Work out the finished part from the listing and answer in its coordinate system (mm). Give positions to 0.01 mm unless a question says otherwise; leave off trailing zeros. Order: outer loops, then holes, each group sorted by start corner. A loop starts at its lowest first (then second) coordinate and runs counter-clockwise, first axis right, second up. Notation, with made-up numbers: (-16.5, 82.5) -> (11.5, 82.5) arc R18 cw to (11.5, 106.5) -> close; hole circle Ø11 at (-8, 38). An arc over 180 degrees is marked (long way). Use a Markdown table: item, result. Add a question column.
```python
from build123d import *

# Parameters (mm, degrees)
SKETCH1_R           = 10
SKETCH1_R_2         = 1.972602619
BOSS_EXTRUDE2_DEPTH = 2
SKETCH5_W           = 5
SKETCH5_H           = 14
CUT_EXTRUDE3_DEPTH  = 3.0000001
SKETCH6_W           = 5
SKETCH6_H           = 14
CUT_EXTRUDE4_DEPTH  = 3.0000001
SKETCH19_R          = 2
CUT_EXTRUDE19_DEPTH = 3.0000001
SKETCH22_R          = 2
CUT_EXTRUDE22_DEPTH = 3.0000001
SKETCH23_R          = 2
CUT_EXTRUDE23_DEPTH = 3.0000001
SKETCH24_R          = 2
CUT_EXTRUDE24_DEPTH = 3.0000001
SKETCH25_W          = 5
SKETCH25_H          = 12
CUT_EXTRUDE25_DEPTH = 3.0000001
CUT_EXTRUDE26_DEPTH = 3.0000001
CUT_EXTRUDE29_DEPTH = 3.0000001
SKETCH20_R          = 2
CUT_EXTRUDE20_DEPTH = 3.0000001
SKETCH30_W          = 181.696441894
SKETCH30_H          = 131.456906608
CUT_EXTRUDE30_DEPTH = 3
SKETCH31_R          = 2
CUT_EXTRUDE31_DEPTH = 2
SKETCH32_W          = 167.461823271
SKETCH32_H          = 37.26795508
CUT_EXTRUDE32_DEPTH = 2
FILLET1_R           = 10
FILLET2_R           = 5


with BuildPart() as part:
    # Sketch1 → Boss-Extrude2 (new body)
    with BuildSketch(Plane.XY):
        with BuildLine():
            Line((-49.4, 97.775402254), (-49.4, 48.775402254))
            Line((-49.4, 48.775402254), (-48.4, 48.775402254))
            Line((-48.4, 48.775402254), (-48.4, 35.775402254))
            Line((-48.4, 35.775402254), (-49.4, 35.775402254))
            Line((-49.4, 35.775402254), (-49.4, 21.775402254))
            Line((-49.4, 21.775402254), (-73.4, 21.775402254))
            Line((-73.4, 21.775402254), (-73.4, -12.924597746))
            Line((-73.4, -12.924597746), (-49.4, -12.924597746))
            Line((-49.4, -12.924597746), (-49.4, -26.924597746))
            Line((-49.4, -26.924597746), (-48.4, -26.924597746))
            Line((-48.4, -26.924597746), (-48.4, -39.924597746))
            Line((-48.4, -39.924597746), (-49.4, -39.924597746))
            Line((-49.4, -39.924597746), (-49.4, -88.924597746))
            Line((-49.4, -88.924597746), (-73.349457369, -88.924597746))
            add(Edge.make_bspline(
                [(-73.349457369, -88.924597746), (-70.502213021, -123.490651401), (3.447241601, -123.490651401), (77.396696223, -123.490651401), (74.549451875, -88.924597746)],
                knots=[3.190793702, 3.190793702, 3.190793702, 4.761590029, 4.761590029, 6.332386355, 6.332386355, 6.332386355], degree=2, weights=[1, 0.707106781, 1, 0.707106781, 1]))
            Line((74.549451875, -88.924597746), (50.599994505, -88.924597746))
            Line((50.599994505, -88.924597746), (50.599994505, -39.924597746))
            Line((50.599994505, -39.924597746), (49.599994505, -39.924597746))
            Line((49.599994505, -39.924597746), (49.599994505, -26.924597746))
            Line((49.599994505, -26.924597746), (50.599994505, -26.924597746))
            Line((50.599994505, -26.924597746), (50.599994505, -12.924597746))
            Line((50.599994505, -12.924597746), (74.599994505, -12.924597746))
            Line((74.599994505, -12.924597746), (74.599994505, 21.775402254))
            Line((74.599994505, 21.775402254), (50.669116659, 21.775402254))
            Line((50.669116659, 21.775402254), (50.669116659, 35.775402254))
            Line((50.669116659, 35.775402254), (49.669116659, 35.775402254))
            Line((49.669116659, 35.775402254), (49.669116659, 48.775402254))
            Line((49.669116659, 48.775402254), (50.669116659, 48.775402254))
            Line((50.669116659, 48.775402254), (50.669116659, 97.775402254))
            Line((50.669116659, 97.775402254), (74.669116659, 97.775402254))
            add(Edge.make_bspline(
                [(74.669116659, 97.775402254), (74.669116659, 132.775402254), (0.587265356, 132.775402254), (-73.494585946, 132.775402254), (-73.494585946, 97.775402254)],
                knots=[3.141592654, 3.141592654, 3.141592654, 4.71238898, 4.71238898, 6.283185307, 6.283185307, 6.283185307], degree=2, weights=[1, 0.707106781, 1, 0.707106781, 1]))
            Line((-73.494585946, 97.775402254), (-49.4, 97.775402254))
        make_face()
        with Locations((0, 72.732378713)):
            Circle(SKETCH1_R, mode=Mode.SUBTRACT)
        with Locations((0, -63.883577786)):
            Circle(SKETCH1_R, mode=Mode.SUBTRACT)
        with Locations((0, 4.424400463)):
            Circle(SKETCH1_R_2, mode=Mode.SUBTRACT)
    extrude(amount=BOSS_EXTRUDE2_DEPTH)

    # Sketch5 → Cut-Extrude3 (cut, through all)
    with BuildSketch(Plane(origin=(0, 0, 0), x_dir=(-1, 0, 0), z_dir=(0, 0, -1))):
        with Locations((46.9, 4.425402254)):
            Rectangle(SKETCH5_W, SKETCH5_H)
    extrude(amount=-CUT_EXTRUDE3_DEPTH, mode=Mode.SUBTRACT)

    # Sketch6 → Cut-Extrude4 (cut, through all)
    with BuildSketch(Plane(origin=(0, 0, 0), x_dir=(-1, 0, 0), z_dir=(0, 0, -1))):
        with Locations((-48.099994505, 4.425402254)):
            Rectangle(SKETCH6_W, SKETCH6_H)
    extrude(amount=-CUT_EXTRUDE4_DEPTH, mode=Mode.SUBTRACT)

    # Sketch19 → Cut-Extrude19 (cut, through all)
    with BuildSketch(Plane(origin=(0, 0, 0), x_dir=(-1, 0, 0), z_dir=(0, 0, -1))):
        with Locations((-56.599994505, 4.425402254)):
            Circle(SKETCH19_R)
    extrude(amount=-CUT_EXTRUDE19_DEPTH, mode=Mode.SUBTRACT)

    # Sketch22 → Cut-Extrude22 (cut, through all)
    with BuildSketch(Plane(origin=(0, 0, 0), x_dir=(-1, 0, 0), z_dir=(0, 0, -1))):
        with Locations((42.4, 81)):
            Circle(SKETCH22_R)
        with Locations((-43.669116659, 81)):
            Circle(SKETCH22_R)
    extrude(amount=-CUT_EXTRUDE22_DEPTH, mode=Mode.SUBTRACT)

    # Sketch23 → Cut-Extrude23 (cut, through all)
    with BuildSketch(Plane.XY.offset(2)):
        with Locations((43.599994505, -81)):
            Circle(SKETCH23_R)
        with Locations((-42.4, -81)):
            Circle(SKETCH23_R)
    extrude(amount=-CUT_EXTRUDE23_DEPTH, mode=Mode.SUBTRACT)

    # Sketch24 → Cut-Extrude24 (cut, through all)
    with BuildSketch(Plane.XY.offset(2)):
        with Locations((-50, -94.924597746)):
            Circle(SKETCH24_R)
        with Locations((50, -94.924597746)):
            Circle(SKETCH24_R)
        with Locations((-50, 103.775402254)):
            Circle(SKETCH24_R)
        with Locations((50, 103.775402254)):
            Circle(SKETCH24_R)
    extrude(amount=-CUT_EXTRUDE24_DEPTH, mode=Mode.SUBTRACT)

    # Sketch25 → Cut-Extrude25 (cut, through all)
    with BuildSketch(Plane(origin=(0, 0, 0), x_dir=(-1, 0, 0), z_dir=(0, 0, -1))):
        with Locations((-28.369116659, 42.275402254)):
            Rectangle(SKETCH25_W, SKETCH25_H)
        with Locations((27.1, 42.275402254)):
            Rectangle(SKETCH25_W, SKETCH25_H)
        with Locations((-28.299994505, -33.424597746)):
            Rectangle(SKETCH25_W, SKETCH25_H)
        with Locations((27.1, -33.424597746)):
            Rectangle(SKETCH25_W, SKETCH25_H)
    extrude(amount=-CUT_EXTRUDE25_DEPTH, mode=Mode.SUBTRACT)

    # Sketch26 → Cut-Extrude26 (cut, through all)
    with BuildSketch(Plane(origin=(0, 0, 0), x_dir=(-1, 0, 0), z_dir=(0, 0, -1))):
        Polygon((24.510151311, 52.075402254), (17.510151311, 52.075402254), (17.510151311, 59.075402254), (13.510151311, 59.075402254), (13.510151311, 66.075402254), (17.510151311, 66.075402254), (17.510151311, 73.075402254), (24.510151311, 73.075402254), (24.510151311, 66.075402254), (28.510151311, 66.075402254), (28.510151311, 59.075402254), (24.510151311, 59.075402254), align=None)
        Polygon((-29.999116659, 59.075402254), (-29.999116659, 66.075402254), (-25.999116659, 66.075402254), (-25.999116659, 73.075402254), (-18.999116659, 73.075402254), (-18.999116659, 66.075402254), (-14.999116659, 66.075402254), (-14.999116659, 59.075402254), (-18.999116659, 59.075402254), (-18.999116659, 52.075402254), (-25.999116659, 52.075402254), (-25.999116659, 59.075402254), align=None)
        Polygon((-19, -69), (-19, -62), (-15, -62), (-15, -55), (-19, -55), (-19, -48), (-26, -48), (-26, -55), (-30, -55), (-30, -62), (-26, -62), (-26, -69), align=None)
        Polygon((24.510151311, -48), (17.510151311, -48), (17.510151311, -55), (13.510151311, -55), (13.510151311, -62), (17.510151311, -62), (17.510151311, -69), (24.510151311, -69), (24.510151311, -62), (28.510151311, -62), (28.510151311, -55), (24.510151311, -55), align=None)
    extrude(amount=-CUT_EXTRUDE26_DEPTH, mode=Mode.SUBTRACT)

    # Sketch28 → Cut-Extrude29 (cut, through all)
    with BuildSketch(Plane(origin=(0, 0, 0), x_dir=(-1, 0, 0), z_dir=(0, 0, -1))):
        with BuildLine():
            Line((28.730883341, 86.928533544), (-30, 86.928533544))
            ThreePointArc((-30, 86.928533544), (-32, 88.928533544), (-30, 90.928533544))
            Line((-30, 90.928533544), (28.730883341, 90.928533544))
            ThreePointArc((28.730883341, 90.928533544), (30.730883341, 88.928533544), (28.730883341, 86.928533544))
        make_face()
    extrude(amount=-CUT_EXTRUDE29_DEPTH, mode=Mode.SUBTRACT)

    # Sketch20 → Cut-Extrude20 (cut, through all)
    with BuildSketch(Plane(origin=(0, 0, 0), x_dir=(-1, 0, 0), z_dir=(0, 0, -1))):
        with Locations((55.4, 4.425402254)):
            Circle(SKETCH20_R)
    extrude(amount=-CUT_EXTRUDE20_DEPTH, mode=Mode.SUBTRACT)

    # Sketch30 → Cut-Extrude30 (cut)
    with BuildSketch(Plane(origin=(0, 0, 0), x_dir=(-1, 0, 0), z_dir=(0, 0, -1))):
        with Locations((-2.534318945, -61.30305105)):
            Rectangle(SKETCH30_W, SKETCH30_H)
    extrude(amount=-CUT_EXTRUDE30_DEPTH, mode=Mode.SUBTRACT)

    # Sketch31 → Cut-Extrude31 (cut)
    with BuildSketch(Plane(origin=(0, 0, 0), x_dir=(-1, 0, 0), z_dir=(0, 0, -1))):
        with Locations((-18.412976441, 45.21289193)):
            Circle(SKETCH31_R)
        with Locations((-18.413659383, 8.47289193)):
            Circle(SKETCH31_R)
        with Locations((18.967023559, 45.21289193)):
            Circle(SKETCH31_R)
        with Locations((18.966340617, 8.47289193)):
            Circle(SKETCH31_R)
    extrude(amount=-CUT_EXTRUDE31_DEPTH, mode=Mode.SUBTRACT)

    # Sketch32 → Cut-Extrude32 (cut)
    with BuildSketch(Plane(origin=(0, 0, 0), x_dir=(-1, 0, 0), z_dir=(0, 0, -1))):
        with Locations((-4.661465148, 116.409379794)):
            Rectangle(SKETCH32_W, SKETCH32_H)
    extrude(amount=-CUT_EXTRUDE32_DEPTH, mode=Mode.SUBTRACT)

    # Fillet1
    fillet1_edges = [part.edges().sort_by_distance(p)[0] for p in [
        (-49.4, 97.775402254, 1),
        (50.669116659, 97.775402254, 1),
    ]]
    fillet(fillet1_edges, radius=FILLET1_R)

    # Fillet2
    fillet2_edges = [part.edges().sort_by_distance(p)[0] for p in [
        (74.599994505, 21.775402254, 1),
        (-73.4, 21.775402254, 1),
    ]]
    fillet(fillet2_edges, radius=FILLET2_R)

    # Mirror1: part across plane


with BuildPart() as part_1:
    add(part.part)
    add(part.part.mirror(Plane(origin=(0, 4.425402254, 0), x_dir=(0, 0, 1), z_dir=(0, -1, 0))))


solid = part_1.part
```
1) Determine the mould class of faces 1 (the flat face through (16, 3, 0)), 2 (the cylindrical face through (47.662, -86.073, 1.014)), 3 (the cylindrical face through (-16.97, 0.29, 0.99)) for opening direction Y: released by +Y, released by -Y, zero draft, split by the parting line, or undercut.
2) Flat-ended cylindrical pins translate along their axes: pin 1 (0.6 mm diameter, centred on y = -54.5, z = 1, fed in from -X); pin 2 (0.6 mm diameter, centred on x = 48, z = 1, fed in from +Y); pin 3 (0.8 mm diameter, centred on x = 50, z = 0.5, fed in from -Y). Find the tip coordinate at first contact, or state that the pin passes through.
3) Straight lines are drawn through the part: line 1 (X direction, y = -64, z = 1.05); line 2 (X direction, y = 45, z = 1.7); line 3 (Y direction, x = -22, z = 0.7). For each, find the intervals that lie inside material, in ascending order.
4) The part is cut by section C-C, the plane z = 1.4. State how many separate pieces and enclosed holes the cut face has, then the cut area to 3 significant figures.
5) The part is cut by section A-A, the plane x = 0. Determine the outline of the cut face in (y, z).
6) The part is cut by section B-B, the plane x = -55.4. Determine the outline of the cut face in (y, z).
A:
| question | item | result |
|---|---|---|
| 1 | face 1 | zero draft |
| 1 | face 2 | released by -Y |
| 1 | face 3 | undercut |
| 2 | pin 1 | x = -49.4 |
| 2 | pin 2 | y = 94.89 |
| 2 | pin 3 | y = -83.42 |
| 3 | line 1 | -49.4 to -24.51, -17.51 to -10, 10 to 19, 26 to 50.67 |
| 3 | line 2 | -48.4 to -29.6, -24.6 to -20.96, -16.98 to 16.42, 20.4 to 25.87, 30.87 to 49.67 |
| 3 | line 3 | -88.92 to -82.08, -78.08 to -64.22, -43.22 to 52.08, 73.08 to 86.93, 90.93 to 97.78 |
| 4 | separate pieces | 1 |
| 4 | enclosed holes | 29 |
| 4 | area | 17,700 mm^2 |
| 5 | outline | (-88.92, 0) -> (-82.08, 0) -> (-82.08, 2) -> (-88.92, 2) -> close; (-78.08, 0) -> (-73.88, 0) -> (-73.88, 2) -> (-78.08, 2) -> close; (-53.88, 0) -> (2.45, 0) -> (2.45, 2) -> (-53.88, 2) -> close; (6.4, 0) -> (62.73, 0) -> (62.73, 2) -> (6.4, 2) -> close; (82.73, 0) -> (86.93, 0) -> (86.93, 2) -> (82.73, 2) -> close; (90.93, 0) -> (97.78, 0) -> (97.78, 2) -> (90.93, 2) -> close |
| 6 | outline | (-12.92, 0) -> (2.43, 0) -> (2.43, 2) -> (-12.92, 2) -> close; (6.43, 0) -> (21.78, 0) -> (21.78, 2) -> (6.43, 2) -> close |
